Geometry: see drawing. Coordinates: mm, zero at the bounding-box minimum. A direction names the side the tool comes from. Round coordinates to 2 decimals unless told otherwise and drop trailing zeros. Loops run counter-clockwise (first coordinate to the right, second up) from the corner with the lowest first, then second, coordinate; pieces in that order, holes last. Notation, with made-up numbers: (4, 34) - (9, 34) arc R28 cw to (9, 70) - close; hole circle Ø9 at (-23.75, 38.5). An arc over 180 degrees is marked (long way). Use CSV: the item, a comma, the result in double quotes.
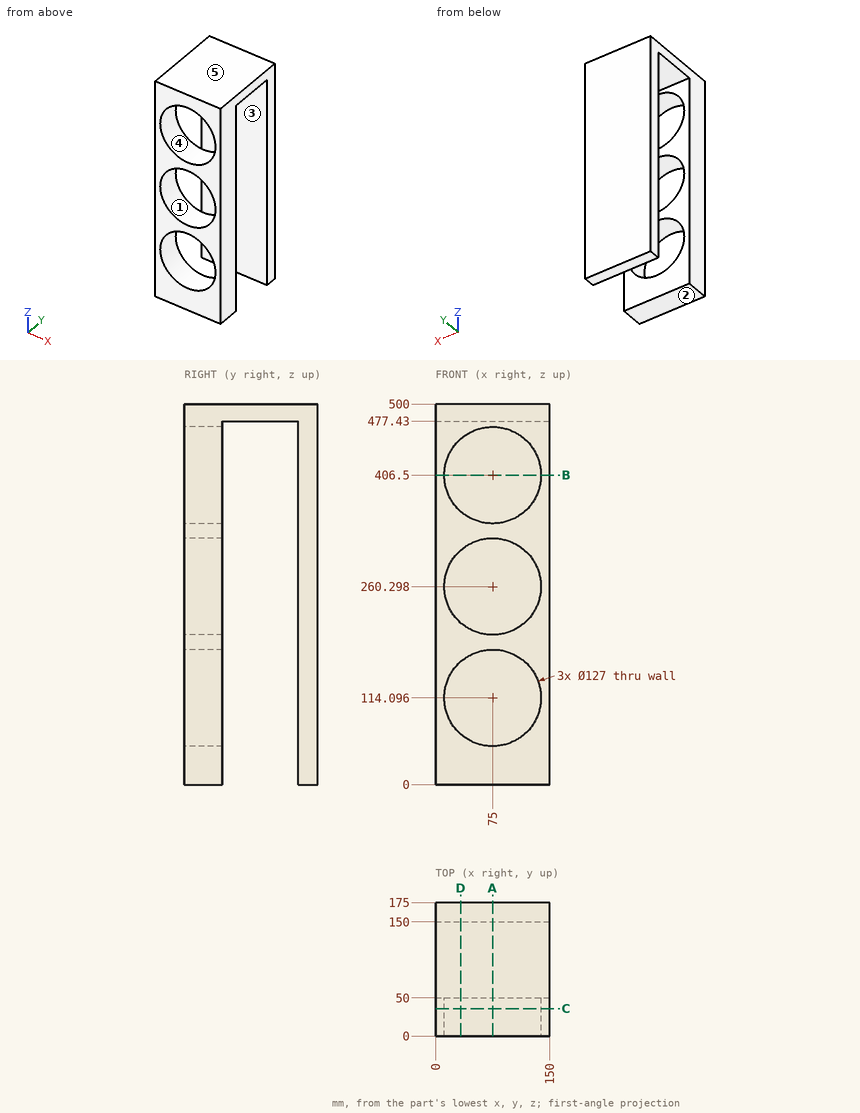
Item 1: Reachability of the marked faces 1, 2 and 3 from +Z, -Z, +X, -X, +Y, -Y: full face, straight path, thin tool, end or side. Return the list, or none.
Final values:
face 1,"-Y"
face 2,"-Z, +X, -X, +Y, -Y"
face 3,"-Z, +X, -X"
Item 2: Mould query, pull axis X, two halves, no side actions, for the marked faces 4 and 5. Classes: released by +X, released by -X, zero draft, split by the parting line, or undercut.
Final values:
face 4,"undercut"
face 5,"zero draft"
Item 3: Section D-D on x = 33. Return the cut outline in (y, z).
Final values:
outline,"(0, 0) - (50, 0) - (50, 66.47) - (0, 66.47) - close; (0, 161.72) - (50, 161.72) - (50, 212.67) - (0, 212.67) - close; (0, 307.92) - (50, 307.92) - (50, 358.87) - (0, 358.87) - close; (0, 454.13) - (50, 454.13) - (50, 477.43) - (150, 477.43) - (150, 0) - (175, 0) - (175, 500) - (0, 500) - close"
Item 4: Section C-C on y = 36. Return the cut outline in (x, z), plus the area to 3 significant figures.
Final values:
outline,"(0, 0) - (150, 0) - (150, 500) - (0, 500) - close; hole circle Ø127 at (75, 114.1); hole circle Ø127 at (75, 260.3); hole circle Ø127 at (75, 406.5)"
area,"37,000 mm²"
Item 5: Section A-A on x = 75. Return the cut outline in (y, z), plus the area to 3 significant figures.
Final values:
outline,"(0, 0) - (50, 0) - (50, 50.6) - (0, 50.6) - close; (0, 177.6) - (50, 177.6) - (50, 196.8) - (0, 196.8) - close; (0, 323.8) - (50, 323.8) - (50, 343) - (0, 343) - close; (0, 470) - (50, 470) - (50, 477.43) - (150, 477.43) - (150, 0) - (175, 0) - (175, 500) - (0, 500) - close"
area,"20,700 mm²"
Item 6: Section B-B on z = 406.5. Return the cut outline in (x, y), plus the area to 3 significant figures.
Final values:
outline,"(0, 0) - (11.5, 0) - (11.5, 50) - (0, 50) - close; (0, 150) - (150, 150) - (150, 175) - (0, 175) - close; (138.5, 0) - (150, 0) - (150, 50) - (138.5, 50) - close"
area,"4,900 mm²"
Item 7: Material intervals for line 1 (Z direction, x = 75, y = 12); line 2 (Y direction, x = 141, z = 85.5); line 3 (Z direction, x = 102.5, y = 34.5) (1 decimal), sorted ascending.
Final values:
line 1,"z = 0 to 50.6, 177.6 to 196.8, 323.8 to 343, 470 to 500"
line 2,"y = 0 to 50, 150 to 175"
line 3,"z = 0 to 56.9, 171.3 to 203.1, 317.5 to 349.3, 463.7 to 500"
Item 8: Pin query (flat end, axial travel): P1, Ø1, axis at x = 59, y = 66.5, coming from the -Z side. Return the tip coordinate at first contact, or that it passes through.
Final values:
P1,"stops at z = 477.43"
